from build123d import *

# Parameters (mm, degrees)
F0_R     = 25.9969
F0_R_2   = 12.50061
F1_DEPTH = 14.9987
F2_R     = 1.524


with BuildPart() as f1:
    # F0 (on Right) → F1 (new body)
    with BuildSketch(Plane.YZ):
        Circle(F0_R)
        Circle(F0_R_2, mode=Mode.SUBTRACT)
    extrude(amount=-F1_DEPTH)

    # F2
    f2_edges = [f1.edges().sort_by_distance(p)[0] for p in [
        (0, -25.9969, 0),
        (0, -12.50061, 0),
        (-14.9987, -25.9969, 0),
        (-14.9987, -12.50061, 0),
    ]]
    fillet(f2_edges, radius=F2_R)


solid = f1.part
Geometry check sheet. Reference: the model listing, model coordinates, mm. Give positions to 0.01 mm unless a question says otherwise; leave off trailing zeros. Write each loop counter-clockwise with the first axis right and the second up, starting at its lowest first coordinate (ties: lowest second). Pieces come first, ordered by that corner, then holes.
1) Go/stop test with flat-tipped pins: pin 1 Ø8 at (x, z) = (-11, 19.5) entering from -Y; pin 2 Ø4 at (x, y) = (-4, 3) entering from +Z; pin 3 Ø1.5 at (x, y) = (-9.5, 5.5) entering from -Z. Record where each tip stops, or that it passes through.
Values follow:
pin 1: stops at y = -20.87
pin 2: stops at z = 25.98
pin 3: stops at z = -25.56
2) Cross-section at C-C (x = -8.5). Record the boundary of the cut face in (y, z), plus the area to 3 significant figures.
Values follow:
outline: circle Ø51.99 at (0, 0); hole circle Ø25 at (0, 0)
area: 1,630 mm2
3) Release check for a two-part mould opening along Z. For faces 1 (the face through (0, 11, -11)), 2 (the face through (-7.416, -2.71, -12.203)), 3 (the face through (-7.416, -5.636, -25.379)) record: released by +Z, released by -Z, zero draft, split by the parting line, or undercut.
Values follow:
face 1: zero draft
face 2: undercut
face 3: split by the parting line
4) Thickness scan on line 1 (Z direction, x = -9.75, y = 0); line 2 (Y direction, x = -12.75, z = -10.5); line 3 (Y direction, x = -7.25, z = -4). Record the ranges inside material, lowest first.
Values follow:
line 1: z = -26 to -12.5, 12.5 to 26
line 2: y = -23.78 to -6.78, 6.78 to 23.78
line 3: y = -25.69 to -11.84, 11.84 to 25.69
5) Cross-section at A-A (z = 0). Record the boundary of the cut face in (x, y).
Values follow:
outline: (-15, -24.47) arc R1.52 ccw to (-13.47, -26) - (-1.52, -26) arc R1.52 ccw to (0, -24.47) - (0, -14.02) arc R1.52 ccw to (-1.52, -12.5) - (-13.47, -12.5) arc R1.52 ccw to (-15, -14.02) - close; (-15, 14.02) arc R1.52 ccw to (-13.47, 12.5) - (-1.52, 12.5) arc R1.52 ccw to (0, 14.02) - (0, 24.47) arc R1.52 ccw to (-1.52, 26) - (-13.47, 26) arc R1.52 ccw to (-15, 24.47) - close
